from build123d import *

# Parameters (mm, degrees)
SKETCH1_R                = 17.272
SKETCH1_R_2              = 9.652
BOSS_EXTRUDE1_DEPTH      = 40.64
BOSS_EXTRUDE2_DEPTH      = 17.78
BOSS_EXTRUDE2_DEPTH_BACK = 17.78
SKETCH3_W                = 34.544
SKETCH3_H                = 40.64
CHAMFER1_SIZE            = 25.24
SKETCH5_R                = 1.75
CUT_EXTRUDE2_DEPTH       = 40.64
SKETCH7_R                = 6.35
CUT_EXTRUDE6_DEPTH       = 30.48
CUT_EXTRUDE7_DEPTH       = 30.48
CUT_EXTRUDE7_DEPTH_BACK  = 30.48
SKETCH8_R                = 3


with BuildPart() as part:
    # Sketch1 → Boss-Extrude1 (new body)
    with BuildSketch(Plane.XY):
        Circle(SKETCH1_R)
        Circle(SKETCH1_R_2, mode=Mode.SUBTRACT)
    extrude(amount=BOSS_EXTRUDE1_DEPTH)

    # Sketch3 → Boss-Extrude2 (add, two sides: drawn at the far end of the back side and taken through both)
    with BuildSketch(Plane(origin=(0, 0, 0), x_dir=(1, 0, 0), z_dir=(0, 1, 0)).offset(-BOSS_EXTRUDE2_DEPTH_BACK)):
        with Locations((0, -60.96)):
            Rectangle(SKETCH3_W, SKETCH3_H)
    extrude(amount=BOSS_EXTRUDE2_DEPTH + BOSS_EXTRUDE2_DEPTH_BACK)

    # Chamfer1
    chamfer1_edges = [part.edges().sort_by_distance(p)[0] for p in [
        (0, -17.78, 81.28),
    ]]
    chamfer(chamfer1_edges, length=CHAMFER1_SIZE)

    # Sketch5 → Cut-Extrude2 (cut)
    with BuildSketch(Plane(origin=(0, 17.78, 0), x_dir=(1, 0, 0), z_dir=(0, 1, 0))):
        with Locations(Location((-9.5, -48.46, 0), (0, 0, 270))):
            Circle(SKETCH5_R)
        with Locations(Location((9.5, -48.46, 0), (0, 0, 270))):
            Circle(SKETCH5_R)
        with Locations(Location((9.5, -73.46, 0), (0, 0, 270))):
            Circle(SKETCH5_R)
        with Locations(Location((-9.5, -73.46, 0), (0, 0, 270))):
            Circle(SKETCH5_R)
    extrude(amount=-CUT_EXTRUDE2_DEPTH, mode=Mode.SUBTRACT)

    # Sketch7 → Cut-Extrude6 (cut)
    with BuildSketch(Plane.XZ.offset(17.78)):
        with Locations(Location((-9.5, 73.46, 0), (0, 0, 270))):
            Circle(SKETCH7_R)
        with Locations(Location((9.5, 73.46, 0), (0, 0, 270))):
            Circle(SKETCH7_R)
        with Locations(Location((-9.5, 48.46, 0), (0, 0, 270))):
            Circle(SKETCH7_R)
        with Locations(Location((9.5, 48.46, 0), (0, 0, 270))):
            Circle(SKETCH7_R)
    extrude(amount=-CUT_EXTRUDE6_DEPTH, mode=Mode.SUBTRACT)

    # Sketch8 → Cut-Extrude7 (cut, two sides: drawn at the far end of the back side and taken through both)
    with BuildSketch(Plane(origin=(0, 0, 0), x_dir=(0, 0, -1), z_dir=(1, 0, 0)).offset(-CUT_EXTRUDE7_DEPTH_BACK)):
        with Locations(Location((-20.32, 0, 0), (0, 0, 180))):
            Circle(SKETCH8_R)
    extrude(amount=CUT_EXTRUDE7_DEPTH + CUT_EXTRUDE7_DEPTH_BACK, mode=Mode.SUBTRACT)


solid = part.part
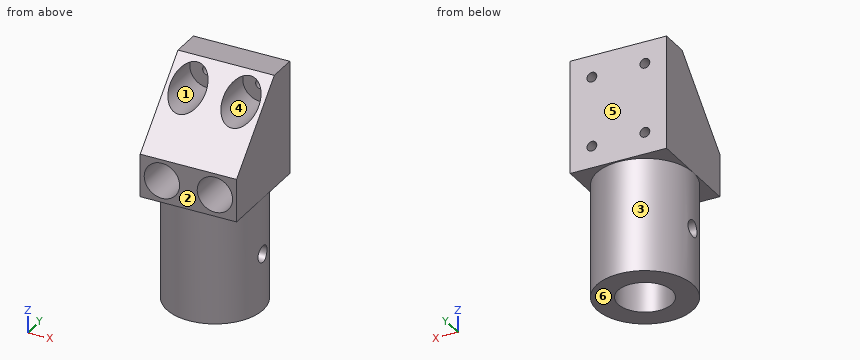
Check sheet for the modelled part. Datum: model origin and axes. Units: mm. Face numbers are marked on the shaded views. A direction names the side the tool comes from. Coordinates: 2 decimals unless noted, no trailing zeros. Loops run counter-clockwise (first coordinate to the right, second up) from the corner with the lowest first, then second, coordinate; pieces in that order, holes last. Notation, with made-up numbers: (56, 31) -> (90, 31) arc R7 ccw to (90, 43) -> close; hole circle Ø6 at (13, 50.25). An arc over 180 degrees is marked (long way). Answer in a Markdown table with one row per item.
1. Sectioned sample at A-A, the plane z = 48.46. Record the boundary of the cut face in (x, y), then the cut area to 3 significant figures.
Check values:
| item | result |
|---|---|
| outline | (-17.27, -17.78) -> (-15.85, -17.78) -> (-15.85, 12.7) -> (-11.25, 12.7) -> (-11.25, 17.78) -> (-17.27, 17.78) -> close; (-7.75, 12.7) -> (-3.15, 12.7) -> (-3.15, -17.78) -> (3.15, -17.78) -> (3.15, 12.7) -> (7.75, 12.7) -> (7.75, 17.78) -> (-7.75, 17.78) -> close; (11.25, 12.7) -> (15.85, 12.7) -> (15.85, -17.78) -> (17.27, -17.78) -> (17.27, 17.78) -> (11.25, 17.78) -> close |
| area | 419 mm2 |
2. Access from +Z, -Z, +X, -X, +Y, -Y to the whole of each face (thin tool, end or side, straight path). Record for the marked faces 1, 2 and 3.
Check values:
| item | result |
|---|---|
| face 1 | -Y |
| face 2 | +Z, -Z, +X, -X, -Y |
| face 3 | -Z |
3. Sectioned sample at B-B, the plane x = 0. Record the boundary of the cut face in (y, z).
Check values:
| item | result |
|---|---|
| outline | (-17.78, 40.64) -> (-17.27, 40.64) -> (-17.27, 0) -> (-9.65, 0) -> (-9.65, 40.64) -> (9.65, 40.64) -> (9.65, 0) -> (17.27, 0) -> (17.27, 40.64) -> (17.78, 40.64) -> (17.78, 81.28) -> (7.46, 81.28) -> (-17.78, 56.04) -> close |
4. Release check for a two-part mould opening along Z. For the marked faces 4, 5 and 6 record: released by +Z, released by -Z, zero draft, split by the parting line, or undercut.
Check values:
| item | result |
|---|---|
| face 4 | undercut |
| face 5 | zero draft |
| face 6 | released by -Z |
5. Sectioned sample at C-C, the plane y = 14. Record the boundary of the cut face in (x, z).
Check values:
| item | result |
|---|---|
| outline | (-17.27, 40.64) -> (-10.12, 40.64) -> (-10.12, 0) -> (10.12, 0) -> (10.12, 40.64) -> (17.27, 40.64) -> (17.27, 81.28) -> (-17.27, 81.28) -> close; hole circle Ø3.5 at (-9.5, 48.46); hole circle Ø3.5 at (-9.5, 73.46); hole circle Ø3.5 at (9.5, 48.46); hole circle Ø3.5 at (9.5, 73.46) |
6. Go/stop test with flat-tipped pins: pin 1 (10 mm diameter, centred on x = -9.5, z = 47.5, fed in from -Y); pin 2 (10 mm diameter, centred on x = 13, y = 8.5, fed in from -Z); pin 3 (8 mm diameter, centred on x = 11.5, z = 14.5, fed in from -Y); pin 4 (3 mm diameter, centred on x = -5.5, y = -2, fed in from +Z). Record where each tip stops, or that it passes through.
Check values:
| item | result |
|---|---|
| pin 1 | stops at y = 12.7 |
| pin 2 | stops at z = 0 |
| pin 3 | stops at y = -15.56 |
| pin 4 | stops at z = 70.29 |
7. Material ranges on line 1 along X through (y, z) = (4.5, 73.46); line 2 along Z through (x, y) = (-11, 6); line 3 along X through (y, z) = (0, 16), recorded low to high. Write a range as [from, to].
Check values:
| item | result |
|---|---|
| line 1 | x = [-17.27, -15.85], [-3.15, 3.15], [15.85, 17.27] |
| line 2 | z = [0, 42.29], [54.63, 67.29], [79.63, 79.82] |
| line 3 | x = [-17.27, -9.65], [9.65, 17.27] |
8. Sectioned sample at D-D, the plane y = -15. Record the boundary of the cut face in (x, z).
Check values:
| item | result |
|---|---|
| outline | (-17.27, 40.64) -> (-8.56, 40.64) -> (-8.56, 0) -> (8.56, 0) -> (8.56, 40.64) -> (17.27, 40.64) -> (17.27, 58.82) -> (-17.27, 58.82) -> close; hole circle Ø12.7 at (-9.5, 48.46); hole circle Ø12.7 at (9.5, 48.46) |
